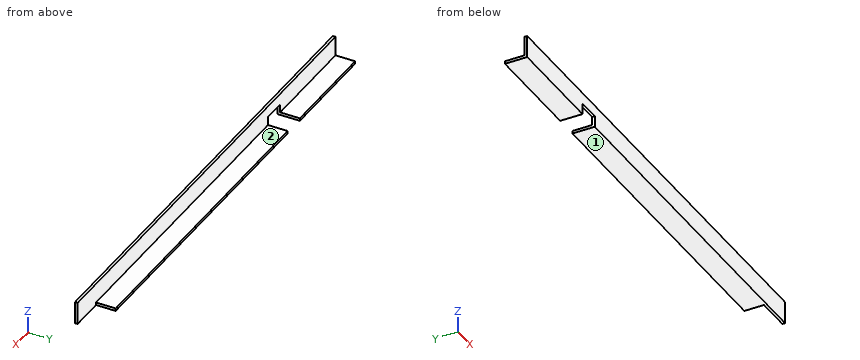
```python
from build123d import *

# Parameters (mm, degrees)
F1_DEPTH = 533.4
F4_DEPTH = 25.4
F6_W     = 22
F6_H     = 3
F7_DEPTH = 38.1


with BuildPart() as f1:
    # F0 (on Right) → F1 (new body)
    with BuildSketch(Plane.YZ):
        Polygon((0, 25), (0, 0), (25, 0), (25, 3), (3, 3), (3, 25), align=None)
    extrude(amount=F1_DEPTH)

    # F3 (on offset) → F4 (cut)
    with BuildSketch(Plane.YZ.offset(114.3)):
        Polygon((0, 12.5), (0, 0), (25, 0), (25, 3), (3, 3), (3, 12.5), align=None)
    extrude(amount=F4_DEPTH, mode=Mode.SUBTRACT)

    # F6 (on offset) → F7 (cut)
    with BuildSketch(Plane.YZ.offset(533.4)):
        with Locations((14, 1.5)):
            Rectangle(F6_W, F6_H)
    extrude(amount=-F7_DEPTH, mode=Mode.SUBTRACT)


solid = f1.part
```
Geometry check sheet. Reference: the model listing, model coordinates, mm. Face numbers are marked on the shaded views. A direction names the side the tool comes from. Round coordinates to 2 decimals unless told otherwise and drop trailing zeros. Loops run counter-clockwise (first coordinate to the right, second up) from the corner with the lowest first, then second, coordinate; pieces in that order, holes last. Notation, with made-up numbers: M 68,27 L 89,27 A18 ccw 89,44 Z; hole C 21.25,59 d11. An arc over 180 degrees is marked long. Return JSON: item names as keys, results as strings. Group by question number.
(1) Section check C-C, the plane z = 20.25. Enter the section's corners in (x, y), and give its area (3 significant figures).
(2) Section check B-B, the plane x = 381.5. Enter the section's corners in (y, z), and give its area (3 significant figures).
(3) Section check A-A, the plane y = 9.5. Enter the section's corners in (x, z).
(4) Set-up check for the marked faces 1 and 2: record each of +Z, -Z, +X, -X, +Y, -Y from which the full face is reachable in a straight line by a thin tool's end or side.
(5) Scan lines: line 1 along X through (y, z) = (2.25, 6.75); line 2 along Z through (x, y) = (163.5, 21.25). Record each from-to range of solid material in increasing order. Write a range as [from, to].
(6) Go/stop test with flat-tipped pins: pin 1 (0.9 mm diameter, centred on x = 129, y = 2, fed in from -Z); pin 2 (7.5 mm diameter, centred on x = 176, z = 18.5, fed in from +Y); pin 3 (10 mm diameter, centred on y = 11, z = 5.5, fed in from +X). Record where each tip stops, or that it passes through.
Data:
{
 "1": {"outline": "M 0,0 L 533.4,0 L 533.4,3 L 0,3 Z", "area": "1,600 mm²"},
 "2": {"outline": "M 0,0 L 25,0 L 25,3 L 3,3 L 3,25 L 0,25 Z", "area": "141 mm²"},
 "3": {"outline": "M 0,0 L 114.3,0 L 114.3,3 L 0,3 Z; M 139.7,0 L 495.3,0 L 495.3,3 L 139.7,3 Z"},
 "4": {"face 1": "-Z, +X, -X, +Y, -Y", "face 2": "+Z, +X, -X, +Y"},
 "5": {"line 1": "[0, 114.3], [139.7, 533.4]", "line 2": "[0, 3]"},
 "6": {"pin 1": "z = 12.5", "pin 2": "y = 3", "pin 3": "x = 495.3"}
}
